Can you work these out from the model? Positions are in its coordinate system, mm. Face numbers are marked on the shaded views. A direction names the side the tool comes from. Give positions to 0.01 mm unless a question says otherwise; leave off trailing zeros. Loops run counter-clockwise (first coordinate to the right, second up) from the corner with the lowest first, then second, coordinate; pieces in that order, holes last. Notation, with made-up numbers: (66, -6) - (100, -6) arc R31 ccw to (100, 19) - close; hole circle Ø8 at (-24.5, 0.5). An arc over 180 degrees is marked (long way). Answer in a Markdown table with one row per item.
from build123d import *

# Parameters (mm, degrees)
F3_W          = 7.8
F3_H          = 10
F3_W_2        = 5.4
F3_H_2        = 2.6
F4_DEPTH      = 7.8
F7_DEPTH      = 3.8
F7_DEPTH_BACK = 3.8
F8_W          = 5.4
F8_H          = 2.6
F9_DEPTH      = 3.9
F10_W         = 1.4347932888
F10_H         = 7.6
F11_DEPTH     = 3.9
F13_DEPTH     = 10.001
F14_T1_DEPTH  = 22.8584149398


# Not quite as in the source:
# - a fillet or chamfer that OpenCascade refuses, or shapes differently, is made with other operations: its cross-section is extruded or revolved along the edge and cut away or added


with BuildPart() as f4:
    # F3 (on Top) → F4 (new body)
    with BuildSketch(Plane.XY):
        Rectangle(F3_W, F3_H)
        Rectangle(F3_W_2, F3_H_2, mode=Mode.SUBTRACT)
        Rectangle(F3_W_2, F3_H_2)
    extrude(amount=F4_DEPTH)

    # F6 (on offset) → F7 (cut, two sides)
    with BuildSketch(Plane.XZ) as f7_sk:
        with BuildLine():
            ThreePointArc((0, 1.2), (1.9091883092, 1.9908116908), (2.7, 3.9))
            ThreePointArc((2.7, 3.9), (1.9091883092, 5.8091883092), (0, 6.6))
            Line((0, 6.6), (0, 3.9))
            Line((0, 3.9), (0, 1.2))
        make_face()
        with BuildLine():
            Line((0, 3.9), (0, 6.6))
            ThreePointArc((0, 6.6), (-2.7, 3.9), (0, 1.2))
            Line((0, 1.2), (0, 3.9))
        make_face()
    extrude(amount=-F7_DEPTH, mode=Mode.SUBTRACT)
    extrude(f7_sk.sketch, amount=F7_DEPTH_BACK, mode=Mode.SUBTRACT)

    # F8 (on face) → F9 (cut)
    with BuildSketch(Plane.XY.offset(7.8)):
        Rectangle(F8_W, F8_H)
    extrude(amount=-F9_DEPTH, mode=Mode.SUBTRACT)

    # F10 (on face) → F11 (cut)
    with BuildSketch(Plane.XY.offset(7.8)):
        Rectangle(F10_W, F10_H)
    extrude(amount=-F11_DEPTH, mode=Mode.SUBTRACT)

    # F12 (on face) → F13 (cut, through all)
    with BuildSketch(Plane.XZ.offset(5)):
        with BuildLine():
            ThreePointArc((0, 2.4), (1.0606601718, 2.8393398282), (1.5, 3.9))
            ThreePointArc((1.5, 3.9), (1.0606601718, 4.9606601718), (0, 5.4))
            Line((0, 5.4), (0, 3.9))
            Line((0, 3.9), (0, 2.4))
        make_face()
        with BuildLine():
            Line((0, 3.9), (0, 5.4))
            ThreePointArc((0, 5.4), (-1.5, 3.9), (0, 2.4))
            Line((0, 2.4), (0, 3.9))
        make_face()
    extrude(amount=-F13_DEPTH, mode=Mode.SUBTRACT)

    # F14: chamfer of 2.5 on 4 edges, made by hand

    # F14_s2 → F14_t1 (cut)
    with BuildSketch(Plane.XZ.offset(-11.4292074699)):
        Polygon((-1.4, 7.8), (-3.9, 5.3), (-3.9, 7.8), align=None)
        Polygon((-1.4, 0), (-3.9, 2.5), (-3.9, 0), align=None)
        Polygon((3.9, 2.5), (1.4, 0), (3.9, 0), align=None)
        Polygon((3.9, 5.3), (1.4, 7.8), (3.9, 7.8), align=None)
    extrude(amount=F14_T1_DEPTH, mode=Mode.SUBTRACT)


solid = f4.part
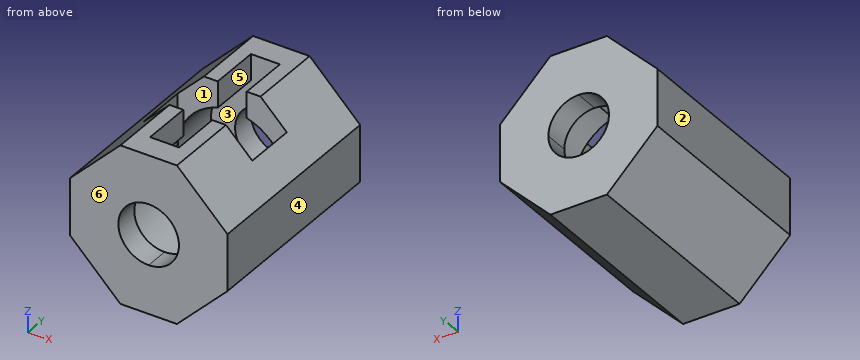
Q1. If we mould it in two halves opening along Y, with no side actions, what happens to the marked faces 3, 4, 5 and 6? For each: released by +Y, released by -Y, zero draft, split by the parting line, or undercut.
Checked values:
| item | result |
|---|---|
| face 3 | undercut |
| face 4 | zero draft |
| face 5 | undercut |
| face 6 | released by -Y |
Q2. For pin 1 (3 mm diameter, centred on y = 1.5, z = 6.5, fed in from +X); pin 2 (1 mm diameter, centred on y = 0, z = 1, fed in from +X); pin 3 (1.4 mm diameter, centred on y = -2, z = 7.5, fed in from +X); pin 4 (0.6 mm diameter, centred on y = 3, z = 7, fed in from -X), each with a flat end and sliding along its axis, tell me the tip position at first contact or that it passes through.
Checked values:
| item | result |
|---|---|
| pin 1 | stops at x = 3.9 |
| pin 2 | stops at x = 2.9 |
| pin 3 | stops at x = 2.4 |
| pin 4 | stops at x = -2.5 |
Q3. Imagine slicing it at A-A, the plane z = 7.5. Write out the boundary of the cut face in (x, y), and give its area (3 significant figures).
Checked values:
| item | result |
|---|---|
| outline | (-1.7, -5) - (1.7, -5) - (1.7, -1.3) - (0.72, -1.3) - (0.72, -3.8) - (-0.72, -3.8) - (-0.72, -1.3) - (-1.7, -1.3) - close; (-1.7, 1.3) - (-0.72, 1.3) - (-0.72, 3.8) - (0.72, 3.8) - (0.72, 1.3) - (1.7, 1.3) - (1.7, 5) - (-1.7, 5) - close |
| area | 18.0 mm² |
Q4. Imagine slicing it at D-D, the plane z = 6.25. Write out the boundary of the cut face in (x, y), and give its area (3 significant figures).
Checked values:
| item | result |
|---|---|
| outline | (-2.95, -5) - (2.95, -5) - (2.95, 5) - (-2.95, 5) - close; hole (-2.7, -1.3) - (-1.33, -1.3) - (-1.33, -3.8) - (1.33, -3.8) - (1.33, -1.3) - (2.7, -1.3) - (2.7, 1.3) - (1.33, 1.3) - (1.33, 3.8) - (-1.33, 3.8) - (-1.33, 1.3) - (-2.7, 1.3) - close |
| area | 31.7 mm² |
Q5. If I drill on line 1 (Y direction, x = -2.5, z = 5.5); line 2 (Y direction, x = 2.5, z = 3.5); line 3 (X direction, y = -1.5, z = 1.5), over which ranges is the centre line in solid material (lowest first)? Write a range as [from, to].
Checked values:
| item | result |
|---|---|
| line 1 | y = [-5, -1.3], [1.3, 5] |
| line 2 | y = [-5, -3.8], [3.8, 5] |
| line 3 | x = [-2.9, -1.24], [1.24, 2.9] |
Q6. On a 3-axis mill with a long thin cutter (end or side, diameter ignored), from which of +Z, -Z, +X, -X, +Y, -Y can I reach the whole of each face in a straight line? I mean the marked faces 1 and 2. Say none if no direction works.
Checked values:
| item | result |
|---|---|
| face 1 | +Z |
| face 2 | +Z, -Z, -X, +Y, -Y |
Q7. Imagine slicing it at B-B, the plane y = -1.75. Write out the boundary of the cut face in (x, z).
Checked values:
| item | result |
|---|---|
| outline | (-3.9, 2.5) - (-1.4, 0) - (1.4, 0) - (3.9, 2.5) - (3.9, 5.3) - (1.4, 7.8) - (0.72, 7.8) - (0.72, 6.5) arc R2.7 cw (long way) to (-0.72, 6.5) - (-0.72, 7.8) - (-1.4, 7.8) - (-3.9, 5.3) - close |
Q8. Imagine slicing it at C-C, the plane x = -1. Write out the boundary of the cut face in (y, z), and give its area (3 significant figures).
Checked values:
| item | result |
|---|---|
| outline | (-5, 0) - (5, 0) - (5, 2.78) - (3.8, 2.78) - (3.8, 1.39) - (-3.8, 1.39) - (-3.8, 2.78) - (-5, 2.78) - close; (-5, 5.02) - (-3.8, 5.02) - (-3.8, 6.41) - (-1.3, 6.41) - (-1.3, 7.8) - (-5, 7.8) - close; (1.3, 6.41) - (3.8, 6.41) - (3.8, 5.02) - (5, 5.02) - (5, 7.8) - (1.3, 7.8) - close |
| area | 30.9 mm² |
